Can you work these out from the model? Positions are in its coordinate system, mm. A direction names the side the tool comes from. Coordinates: 2 decimals unless noted, no trailing zeros. Order: outer loops, then holes, each group sorted by start corner. A loop starts at its lowest first (then second) coordinate and runs counter-clockwise, first axis right, second up. Notation, with made-up numbers: (-16, 19.25) -> (22, 19.25) arc R15 cw to (22, 43.25) -> close; hole circle Ø4 at (38.5, -22). An arc over 180 degrees is marked (long way). Use a Markdown table: item, result. Add a question column.
1. Suppose I cut it at C-C, the plane x = 33. List the corners of the cut face in (y, z) for me.
2. For faces 1 (the flat face through (22, 16, 0)), 2 (the flat face through (22, 15, 0)), which set-ups out of +Z, -Z, +X, -X, +Y, -Y let a thin tool reach every point of the face, with its end or its side?
3. Suppose I cut it at A-A, the plane z = 4. List the corners of the cut face in (x, y) for me.
4. We'd pull the mould along Z, two halves only. Please class faces 3 (the cylindrical face through (101.586, 11.507, 0.07)), 4 (the flat face through (49.8, 15.2, -5)), 5 (the flat face through (82, 12, 0)): pulls with the +Z half, pulls with the -Z half, needs draft (parallel to the pull), parting line crosses it, or undercut.
5. If I drill on line 1 along Z through (x, y) = (0, 15.8); line 2 along Y through (x, z) = (85.5, 3); line 3 along Y through (x, z) = (15, 3.25), over which ranges is the centre line in solid material (lowest first)? Write a range as from..to.
6. For pin 1 Ø2 at (x, z) = (31.5, -1) entering from -Y; pin 2 Ø3.5 at (x, z) = (100, 0) entering from +Y; pin 3 Ø2 at (y, z) = (15, 2) entering from +X, each with a flat end and sliding along its axis, tell me the tip position at first contact or that it passes through.
7. Suppose I cut it at B-B, the plane y = 13.2. List the corners of the cut face in (x, z) for me.
```python
from build123d import *

# Parameters (mm, degrees)
F1_DEPTH = 5
F3_D     = 3.175
F4_R     = 4.5


with BuildPart() as f1:
    # F0 (on Top) → F1 (new body, symmetric)
    with BuildSketch(Plane.XY):
        with BuildLine():
            Line((-5, 16), (-5, 15))
            Line((-5, 15), (49.196152, 15))
            ThreePointArc((49.196152, 15), (49.97261, 14.897777), (50.696152, 14.598076))
            Line((50.696152, 14.598076), (56, 11.535898))
            ThreePointArc((56, 11.535898), (56.964724, 11.136297), (58, 11))
            Line((58, 11), (105, 11))
            Line((105, 11), (105, 12))
            Line((105, 12), (58, 12))
            ThreePointArc((58, 12), (57.223543, 12.102223), (56.5, 12.401924))
            Line((56.5, 12.401924), (51.196152, 15.464102))
            ThreePointArc((51.196152, 15.464102), (50.231429, 15.863703), (49.196152, 16))
            Line((49.196152, 16), (-5, 16))
        make_face()
    extrude(amount=F1_DEPTH, both=True)

    # F3 (through all)
    with Locations(Plane.XZ):
        with Locations((0, 0), (100, 0)):
            Hole(F3_D / 2)

    # F4
    f4_edges = [f1.edges().sort_by_distance(p)[0] for p in [
        (105, 11.5, 5),
        (105, 11.5, -5),
        (-5, 15.5, 5),
        (-5, 15.5, -5),
    ]]
    fillet(f4_edges, radius=F4_R)


solid = f1.part
```
Worked out:
| question | item | result |
|---|---|---|
| 1 | outline | (15, -5) -> (16, -5) -> (16, 5) -> (15, 5) -> close |
| 2 | face 1 | +Z, -Z, +X, -X, +Y |
| 2 | face 2 | +Z, -Z, -X, -Y |
| 3 | outline | (-3.33, 15) -> (49.2, 15) arc R3 cw to (50.7, 14.6) -> (56, 11.54) arc R4 ccw to (58, 11) -> (103.33, 11) -> (103.33, 12) -> (58, 12) arc R3 cw to (56.5, 12.4) -> (51.2, 15.46) arc R4 ccw to (49.2, 16) -> (-3.33, 16) -> close |
| 4 | face 3 | undercut |
| 4 | face 4 | pulls with the -Z half |
| 4 | face 5 | needs draft |
| 5 | line 1 | z = -5..-1.59, 1.59..5 |
| 5 | line 2 | y = 11..12 |
| 5 | line 3 | y = 15..16 |
| 6 | pin 1 | stops at y = 15 |
| 6 | pin 2 | stops at y = 12 |
| 6 | pin 3 | stops at x = 53.73 |
| 7 | outline | (53.12, -5) -> (55.12, -5) -> (55.12, 5) -> (53.12, 5) -> close |
